Autodesk Inventor part; units mm, degrees
ref_plane "YZ Plane" through (0, 0, 0) normal (1, 0, 0) x (0, 1, 0)
ref_plane "XZ Plane" through (0, 0, 0) normal (0, 1, 0) x (-1, 0, 0)
ref_plane "XY Plane" through (0, 0, 0) normal (0, 0, 1) x (1, 0, 0)
sketch "Sketch1" plane through (0, 0, 0) normal (0, 0, 1) x (1, 0, 0)
  line L0 (0, 0) -> (0, 12.5096)
  arc A0 (4.5242, 14.5927) -> (0, 12.5096) centre (2.7416, 12.5096) ccw
  arc A1 (6.2274, 6) -> (4.5242, 14.5927) centre (-0.0774, 9.2154) ccw
  line L1 (6.2274, 6) -> (5.6605, 6)
  arc A2 (5.6605, 6) -> (4.1991, 14.2128) centre (-0.0774, 9.2154) ccw
  arc A3 (4.1991, 14.2128) -> (0.5, 12.5096) centre (2.7416, 12.5096) ccw
  line L2 (0.5, 12.5096) -> (0.5, 0)
  line L3 (0, 0) -> (0.5, 0)
  line L4 (7, 9.2154) -> (7, 0)
  point P0 (0.25, 0)
  point P1 (1.595, 15)
  point P2 (5.9439, 6)
  point P3 (6.8649, 10.5915)
  dimension "d0" = 0.5
  dimension "d1" = 15
  dimension "d2" = 6
  dimension "d4" = 7
extrude "Extrusion1" add sketch "Sketch1" along normal mid plane 7
sketch "Sketch2" plane through (0, 0, -3.5) normal (-1, 0, 0) x (0, 0, 1)
  line L0 (2.5, 0) -> (4.5, 0)
  line L1 (4.5, 0) -> (4.5, 0.5)
  line L2 (4.5, 0.5) -> (2.5, 0.5)
  line L3 (2.5, 0.5) -> (2.5, 0)
  line L4 (0, 0) -> (7, 0)
  point P0 (3.5, 0.5)
  point P1 (3.5, 0)
  dimension "d8" = 2
extrude "Extrusion2" add sketch "Sketch2" along normal blind 4.5
fillet "Fillet1" radius 1 2 edges at (-4.5, 0.25, 1) (-4.5, 0.25, -1)
properties part number "Holder_Metal"
Design review of the part built by this model. Coordinates are the model's own, in mm. A direction names the side the tool comes from. Round coordinates to 2 decimals unless told otherwise and drop trailing zeros. Order: outer loops, then holes, each group sorted by start corner. A loop starts at its lowest first (then second) coordinate and runs counter-clockwise, first axis right, second up. Notation, with made-up numbers: (9.25, -32.75) - (56.25, -32.75) arc R17 cw to (56.25, -11.75) - close; hole circle Ø4 at (58, 68.25). An arc over 180 degrees is marked (long way). Return JSON: item names as keys, results as strings.
Q1. Consider section A-A on y = 12.75. Write out the cut boundary in (x, z), plus the area to 3 significant figures.
Computed values:
{"outline": "(0.01, -3.5) - (0.51, -3.5) - (0.51, 3.5) - (0.01, 3.5) - close; (5.47, -3.5) - (6.05, -3.5) - (6.05, 3.5) - (5.47, 3.5) - close", "area": "7.61 mm2"}
Q2. For pin 1 Ø3 at (x, z) = (-3, 2) entering from +Y; pin 2 Ø1 at (y, z) = (10, 0) entering from +X; pin 3 Ø0.6 at (x, z) = (6, -1.5) entering from -Y, all flat-tipped, find the tip position at first contact; note any pin that passes through.
Computed values:
{"pin 1": "stops at y = 0.5", "pin 2": "stops at x = 6.99", "pin 3": "stops at y = 6"}
Q3. Consider section D-D on y = 8. Write out the cut boundary in (x, z).
Computed values:
{"outline": "(0, -3.5) - (0.5, -3.5) - (0.5, 3.5) - (0, 3.5) - close; (6.39, -3.5) - (6.89, -3.5) - (6.89, 3.5) - (6.39, 3.5) - close"}
Q4. Consider section C-C on x = -1. Write out the cut boundary in (y, z), plus the area to 3 significant figures.
Computed values:
{"outline": "(0, -1) - (0.5, -1) - (0.5, 1) - (0, 1) - close", "area": "1.00 mm2"}
Q5. The part is to be moulded in two halves that separate along X. For faces 1 (the cylindrical face through (-4.215, 0.254, 0.699)), 2 (the cylindrical face through (1.555, 14.981, -0.049)), 3 (the cylindrical face through (6.387, 10.43, -0.049)), say which applies: pulls with the +X half, pulls with the -X half, needs draft (parallel to the pull), parting line crosses it, or undercut.
Computed values:
{"face 1": "pulls with the -X half", "face 2": "parting line crosses it", "face 3": "undercut"}
Q6. Consider section B-B on z = -2. Write out the cut boundary in (x, y).
Computed values:
{"outline": "(0, 0) - (0.5, 0) - (0.5, 12.51) arc R2.24 cw to (4.2, 14.21) arc R6.58 cw to (5.66, 6) - (6.23, 6) arc R7.08 ccw to (4.52, 14.59) arc R2.74 ccw to (0, 12.51) - close"}
Q7. Machinability: for faces 4 (the flat face through (0.5, 6, 0)), 5 (the flat face through (-1, 0, 0)), 6 (the flat face through (-2, 0.5, 0)), which of the approach directions +Z, -Z, +X, -X, +Y, -Y give a long, thin tool a straight path to every point of the face, cutting with its end or side? Answer none if there is none.
Computed values:
{"face 4": "+Z, -Z, -Y", "face 5": "+Z, -Z, +X, -X, -Y", "face 6": "+Z, -Z, -X, +Y"}
Q8. Wall thickness on L1, parallel to X at y = 9, z = 2.75; L2, parallel to X at y = 2.5, z = 3; L3, parallel to X at y = 13.5, z = -0.25: over which ranges is each line inside the solid? List them lowest first. Write a range as [from, to].
Computed values:
{"L1": "x = [0, 0.5], [6.5, 7]", "L2": "x = [0, 0.5]", "L3": "x = [0.19, 0.73], [4.91, 5.56]"}
